Work out the finished part from the listing and answer in its coordinate system (mm). Coordinates: 2 decimals unless noted, no trailing zeros. Write each loop counter-clockwise with the first axis right and the second up, starting at its lowest first coordinate (ties: lowest second). Pieces come first, ordered by that corner, then holes. Notation, with made-up numbers: (2, 5) - (37, 5) arc R37 ccw to (37, 43) - close; hole circle Ø5 at (2, 84.5). An arc over 180 degrees is marked (long way). Use one line per item in the form item = value. Start each with the question number.
Item 1: A cutting plane is placed at B-B (z = -0.75). Write down the section's boundary in (x, y).
Item 2: A cutting plane is placed at D-D (x = -15). Write down the section's boundary in (y, z).
Item 3: Consider probe 1 along X at (y, z) = (0.45, -6); probe 2 along X at (y, z) = (1.2, -12.75); probe 3 along Z at (x, y) = (4, 1.8). Determine where each line is inside the solid, lowest interval first.
Item 4: A cutting plane is placed at C-C (z = -10.75). Write down the section's boundary in (x, y), then the cut area to 3 significant figures.
Item 5: A cutting plane is placed at A-A (x = 24). Write down the section's boundary in (y, z), then the cut area to 3 significant figures.
Item 6: Given pin 1 (2 mm diameter, centred on x = 34.5, z = -11.5, fed in from +Y); pin 2 (2.5 mm diameter, centred on x = 1, z = -8, fed in from +Y), each flat-ended and moving along its own axis, determine where each tip first touches the part or whether it passes through.
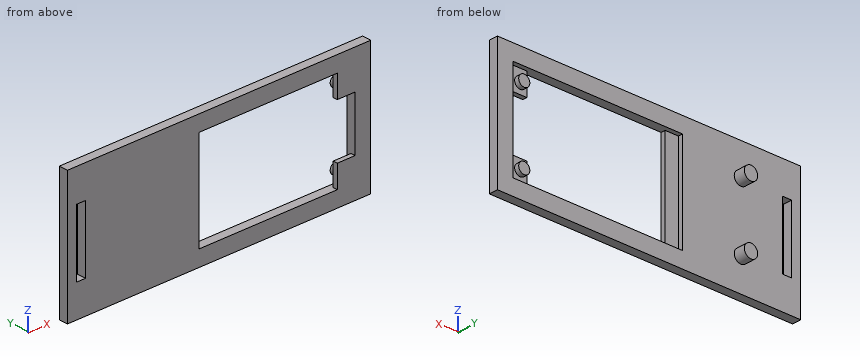
from build123d import *

# Parameters (mm, degrees)
SKETCH1_W             = 68
SKETCH1_H             = 29
BASE_DEPTH            = 2
SKETCH2_R             = 1.5
LEFT_PEG_DEPTH        = 2.5
SKETCH3_R             = 1.5
RIGHT_PEG_DEPTH       = 2.5
SKETCH4_W             = 2
SKETCH4_H             = 14.7
ACCEL_WIRE_HOLE_DEPTH = 2.5
SKETCH5_W             = 38
SKETCH5_H             = 22
OUTER_CUT_DEPTH       = 1
SKETCH6_W             = 31
SKETCH6_H             = 22
INNER_CUT_DEPTH       = 1
SKETCH7_W             = 4
SKETCH7_H             = 12
BETWEEN_PEG_CUT_DEPTH = 1
SKETCH8_R             = 1.25
PEGS_DEPTH            = 1


with BuildPart() as part:
    # Sketch1 → base (new body)
    with BuildSketch(Plane(origin=(0, 0, 0), x_dir=(1, 0, 0), z_dir=(0, 1, 0))):
        with Locations((6.444444444, 2.555555556)):
            Rectangle(SKETCH1_W, SKETCH1_H)
    extrude(amount=BASE_DEPTH)

    # Sketch2 → left peg (add)
    with BuildSketch(Plane(origin=(0, 2, 0), x_dir=(1, 0, 0), z_dir=(0, 1, 0))):
        with Locations(Location((-14.155555556, -4.794444444, 0), (0, 0, 270))):
            Circle(SKETCH2_R)
    extrude(amount=LEFT_PEG_DEPTH)

    # Sketch3 → right peg (add)
    with BuildSketch(Plane(origin=(0, 2, 0), x_dir=(1, 0, 0), z_dir=(0, 1, 0))):
        with Locations(Location((-14.155555556, 9.905555556, 0), (0, 0, 270))):
            Circle(SKETCH3_R)
    extrude(amount=RIGHT_PEG_DEPTH)

    # Sketch4 → accel wire hole (cut)
    with BuildSketch(Plane(origin=(0, 2, 0), x_dir=(1, 0, 0), z_dir=(0, 1, 0))):
        with Locations((-24.505555556, 2.555555556)):
            Rectangle(SKETCH4_W, SKETCH4_H)
    extrude(amount=-ACCEL_WIRE_HOLE_DEPTH, mode=Mode.SUBTRACT)

    # Sketch5 → outer cut (cut)
    with BuildSketch(Plane(origin=(0, 2, 0), x_dir=(1, 0, 0), z_dir=(0, 1, 0))):
        with Locations((17.944444444, 2.555555556)):
            Rectangle(SKETCH5_W, SKETCH5_H)
    extrude(amount=-OUTER_CUT_DEPTH, mode=Mode.SUBTRACT)

    # Sketch6 → inner cut (cut)
    with BuildSketch(Plane(origin=(0, 1, 0), x_dir=(1, 0, 0), z_dir=(0, 1, 0))):
        with Locations((17.444444444, 2.555555556)):
            Rectangle(SKETCH6_W, SKETCH6_H)
    extrude(amount=-INNER_CUT_DEPTH, mode=Mode.SUBTRACT)

    # Sketch7 → between peg cut (cut)
    with BuildSketch(Plane(origin=(0, 1, 0), x_dir=(1, 0, 0), z_dir=(0, 1, 0))):
        with Locations((34.944444444, 2.555555556)):
            Rectangle(SKETCH7_W, SKETCH7_H)
    extrude(amount=-BETWEEN_PEG_CUT_DEPTH, mode=Mode.SUBTRACT)

    # Sketch8 → pegs (add)
    with BuildSketch(Plane(origin=(0, 1, 0), x_dir=(1, 0, 0), z_dir=(0, 1, 0))):
        with Locations(Location((34.414871673, 10.805555556, 0), (0, 0, 270))):
            Circle(SKETCH8_R)
        with Locations(Location((34.414871673, -5.694444444, 0), (0, 0, 270))):
            Circle(SKETCH8_R)
    extrude(amount=PEGS_DEPTH)


solid = part.part
Answer:
q1.outline = (-27.56, 0) - (-25.51, 0) - (-25.51, 2) - (-27.56, 2) - close; (-23.51, 0) - (1.94, 0) - (1.94, 1) - (-1.06, 1) - (-1.06, 2) - (-23.51, 2) - close; (36.94, 0) - (40.44, 0) - (40.44, 2) - (36.94, 2) - close
q2.outline = (0, -17.06) - (2, -17.06) - (2, -11.15) - (4.5, -11.15) - (4.5, -8.67) - (2, -8.67) - (2, 3.55) - (4.5, 3.55) - (4.5, 6.03) - (2, 6.03) - (2, 11.94) - (0, 11.94) - close
q3.probe_1 = -27.56 to -25.51, -23.51 to 1.94, 36.94 to 40.44
q3.probe_2 = -27.56 to -1.06, 36.94 to 40.44
q3.probe_3 = -17.06 to -13.56, 8.44 to 11.94
q4.outline = (-27.56, 0) - (1.94, 0) - (1.94, 1) - (-1.06, 1) - (-1.06, 2) - (-12.92, 2) - (-12.92, 4.5) - (-15.4, 4.5) - (-15.4, 2) - (-27.56, 2) - close; (32.94, 0) - (40.44, 0) - (40.44, 2) - (36.94, 2) - (36.94, 1) - (35.66, 1) - (35.66, 2) - (33.17, 2) - (33.17, 1) - (32.94, 1) - close
q4.area = 75.7 mm²
q5.outline = (0, -17.06) - (2, -17.06) - (2, -13.56) - (0, -13.56) - close; (0, 8.44) - (2, 8.44) - (2, 11.94) - (0, 11.94) - close
q5.area = 14.0 mm²
q6.pin_1 = 2
q6.pin_2 = 1
